```python
from build123d import *

# Parameters (mm, degrees)
SKETCH1_W           = 107.95
SKETCH1_H           = 101.6
BOSS_EXTRUDE1_DEPTH = 3.175
CUT_EXTRUDE1_REACH  = 5.175
SKETCH2_R           = 15.24
CUT_EXTRUDE2_REACH  = 5.175
SKETCH3_R           = 1.5875
CUT_EXTRUDE3_REACH  = 5.175
SKETCH4_R           = 2.1971
FILLET1_R           = 2.54
CUT_EXTRUDE4_DEPTH  = 4.175
FILLET3_R           = 0.0635


with BuildPart() as part:
    # Sketch1 → Boss-Extrude1 (new body)
    with BuildSketch(Plane.XY):
        with Locations((-16.095613336, 62.506086957)):
            Rectangle(SKETCH1_W, SKETCH1_H)
    extrude(amount=BOSS_EXTRUDE1_DEPTH)

    # Sketch2 → Cut-Extrude1 (cut, up to next)
    with BuildSketch(Plane.XY.offset(3.175), mode=Mode.PRIVATE) as cut_extrude1_sk1:
        with Locations((-16.095613336, 62.506086957)):
            Circle(SKETCH2_R)
    cut_extrude1_tool1 = extrude(cut_extrude1_sk1.sketch, amount=-CUT_EXTRUDE1_REACH, mode=Mode.PRIVATE) & part.part
    add(cut_extrude1_tool1.solids().sort_by_distance((-16.095613, 62.506087, 3.175))[0], mode=Mode.SUBTRACT)
    # Sketch2 → Cut-Extrude1 (cut, up to next)
    with BuildSketch(Plane.XY.offset(3.175), mode=Mode.PRIVATE) as cut_extrude1_sk2:
        with Locations((16.596179657, 32.989293963)):
            Circle(SKETCH2_R)
    cut_extrude1_tool2 = extrude(cut_extrude1_sk2.sketch, amount=-CUT_EXTRUDE1_REACH, mode=Mode.PRIVATE) & part.part
    add(cut_extrude1_tool2.solids().sort_by_distance((16.59618, 32.989294, 3.175))[0], mode=Mode.SUBTRACT)
    # Sketch2 → Cut-Extrude1 (cut, up to next)
    with BuildSketch(Plane.XY.offset(3.175), mode=Mode.PRIVATE) as cut_extrude1_sk3:
        with Locations((16.596179657, 92.02287995)):
            Circle(SKETCH2_R)
    cut_extrude1_tool3 = extrude(cut_extrude1_sk3.sketch, amount=-CUT_EXTRUDE1_REACH, mode=Mode.PRIVATE) & part.part
    add(cut_extrude1_tool3.solids().sort_by_distance((16.59618, 92.02288, 3.175))[0], mode=Mode.SUBTRACT)
    # Sketch2 → Cut-Extrude1 (cut, up to next)
    with BuildSketch(Plane.XY.offset(3.175), mode=Mode.PRIVATE) as cut_extrude1_sk4:
        with Locations((-48.787406329, 92.02287995)):
            Circle(SKETCH2_R)
    cut_extrude1_tool4 = extrude(cut_extrude1_sk4.sketch, amount=-CUT_EXTRUDE1_REACH, mode=Mode.PRIVATE) & part.part
    add(cut_extrude1_tool4.solids().sort_by_distance((-48.787406, 92.02288, 3.175))[0], mode=Mode.SUBTRACT)
    # Sketch2 → Cut-Extrude1 (cut, up to next)
    with BuildSketch(Plane.XY.offset(3.175), mode=Mode.PRIVATE) as cut_extrude1_sk5:
        with Locations((-48.787406329, 32.989293963)):
            Circle(SKETCH2_R)
    cut_extrude1_tool5 = extrude(cut_extrude1_sk5.sketch, amount=-CUT_EXTRUDE1_REACH, mode=Mode.PRIVATE) & part.part
    add(cut_extrude1_tool5.solids().sort_by_distance((-48.787406, 32.989294, 3.175))[0], mode=Mode.SUBTRACT)

    # Sketch3 → Cut-Extrude2 (cut, up to next)
    with BuildSketch(Plane.XY.offset(3.175), mode=Mode.PRIVATE) as cut_extrude2_sk1:
        with Locations((-31.186104332, 109.624181947)):
            Circle(SKETCH3_R)
    cut_extrude2_tool1 = extrude(cut_extrude2_sk1.sketch, amount=-CUT_EXTRUDE2_REACH, mode=Mode.PRIVATE) & part.part
    add(cut_extrude2_tool1.solids().sort_by_distance((-31.186104, 109.624182, 3.175))[0], mode=Mode.SUBTRACT)
    # Sketch3 → Cut-Extrude2 (cut, up to next)
    with BuildSketch(Plane.XY.offset(3.175), mode=Mode.PRIVATE) as cut_extrude2_sk2:
        with Locations((-66.388708326, 74.421577952)):
            Circle(SKETCH3_R)
    cut_extrude2_tool2 = extrude(cut_extrude2_sk2.sketch, amount=-CUT_EXTRUDE2_REACH, mode=Mode.PRIVATE) & part.part
    add(cut_extrude2_tool2.solids().sort_by_distance((-66.388708, 74.421578, 3.175))[0], mode=Mode.SUBTRACT)
    # Sketch3 → Cut-Extrude2 (cut, up to next)
    with BuildSketch(Plane.XY.offset(3.175), mode=Mode.PRIVATE) as cut_extrude2_sk3:
        with Locations((-1.00512234, 109.624181947)):
            Circle(SKETCH3_R)
    cut_extrude2_tool3 = extrude(cut_extrude2_sk3.sketch, amount=-CUT_EXTRUDE2_REACH, mode=Mode.PRIVATE) & part.part
    add(cut_extrude2_tool3.solids().sort_by_distance((-1.005122, 109.624182, 3.175))[0], mode=Mode.SUBTRACT)
    # Sketch3 → Cut-Extrude2 (cut, up to next)
    with BuildSketch(Plane.XY.offset(3.175), mode=Mode.PRIVATE) as cut_extrude2_sk4:
        with Locations((34.197481654, 74.421577952)):
            Circle(SKETCH3_R)
    cut_extrude2_tool4 = extrude(cut_extrude2_sk4.sketch, amount=-CUT_EXTRUDE2_REACH, mode=Mode.PRIVATE) & part.part
    add(cut_extrude2_tool4.solids().sort_by_distance((34.197482, 74.421578, 3.175))[0], mode=Mode.SUBTRACT)
    # Sketch3 → Cut-Extrude2 (cut, up to next)
    with BuildSketch(Plane.XY.offset(3.175), mode=Mode.PRIVATE) as cut_extrude2_sk5:
        with Locations((-31.186104332, 15.387991966)):
            Circle(SKETCH3_R)
    cut_extrude2_tool5 = extrude(cut_extrude2_sk5.sketch, amount=-CUT_EXTRUDE2_REACH, mode=Mode.PRIVATE) & part.part
    add(cut_extrude2_tool5.solids().sort_by_distance((-31.186104, 15.387992, 3.175))[0], mode=Mode.SUBTRACT)
    # Sketch3 → Cut-Extrude2 (cut, up to next)
    with BuildSketch(Plane.XY.offset(3.175), mode=Mode.PRIVATE) as cut_extrude2_sk6:
        with Locations((-66.388708326, 50.590595961)):
            Circle(SKETCH3_R)
    cut_extrude2_tool6 = extrude(cut_extrude2_sk6.sketch, amount=-CUT_EXTRUDE2_REACH, mode=Mode.PRIVATE) & part.part
    add(cut_extrude2_tool6.solids().sort_by_distance((-66.388708, 50.590596, 3.175))[0], mode=Mode.SUBTRACT)
    # Sketch3 → Cut-Extrude2 (cut, up to next)
    with BuildSketch(Plane.XY.offset(3.175), mode=Mode.PRIVATE) as cut_extrude2_sk7:
        with Locations((-1.00512234, 15.387991966)):
            Circle(SKETCH3_R)
    cut_extrude2_tool7 = extrude(cut_extrude2_sk7.sketch, amount=-CUT_EXTRUDE2_REACH, mode=Mode.PRIVATE) & part.part
    add(cut_extrude2_tool7.solids().sort_by_distance((-1.005122, 15.387992, 3.175))[0], mode=Mode.SUBTRACT)
    # Sketch3 → Cut-Extrude2 (cut, up to next)
    with BuildSketch(Plane.XY.offset(3.175), mode=Mode.PRIVATE) as cut_extrude2_sk8:
        with Locations((34.197481654, 50.590595961)):
            Circle(SKETCH3_R)
    cut_extrude2_tool8 = extrude(cut_extrude2_sk8.sketch, amount=-CUT_EXTRUDE2_REACH, mode=Mode.PRIVATE) & part.part
    add(cut_extrude2_tool8.solids().sort_by_distance((34.197482, 50.590596, 3.175))[0], mode=Mode.SUBTRACT)
    # Sketch3 → Cut-Extrude2 (cut, up to next)
    with BuildSketch(Plane.XY.offset(3.175), mode=Mode.PRIVATE) as cut_extrude2_sk9:
        with Locations((8.796386664, 62.506086957)):
            Circle(SKETCH3_R)
    cut_extrude2_tool9 = extrude(cut_extrude2_sk9.sketch, amount=-CUT_EXTRUDE2_REACH, mode=Mode.PRIVATE) & part.part
    add(cut_extrude2_tool9.solids().sort_by_distance((8.796387, 62.506087, 3.175))[0], mode=Mode.SUBTRACT)
    # Sketch3 → Cut-Extrude2 (cut, up to next)
    with BuildSketch(Plane.XY.offset(3.175), mode=Mode.PRIVATE) as cut_extrude2_sk10:
        with Locations((-40.987613336, 62.506086957)):
            Circle(SKETCH3_R)
    cut_extrude2_tool10 = extrude(cut_extrude2_sk10.sketch, amount=-CUT_EXTRUDE2_REACH, mode=Mode.PRIVATE) & part.part
    add(cut_extrude2_tool10.solids().sort_by_distance((-40.987613, 62.506087, 3.175))[0], mode=Mode.SUBTRACT)

    # Sketch4 → Cut-Extrude3 (cut, up to next)
    with BuildSketch(Plane.XY.offset(3.175), mode=Mode.PRIVATE) as cut_extrude3_sk1:
        with Locations((-16.095613336, 100.606086957)):
            Circle(SKETCH4_R)
    cut_extrude3_tool1 = extrude(cut_extrude3_sk1.sketch, amount=-CUT_EXTRUDE3_REACH, mode=Mode.PRIVATE) & part.part
    add(cut_extrude3_tool1.solids().sort_by_distance((-16.095613, 100.606087, 3.175))[0], mode=Mode.SUBTRACT)
    # Sketch4 → Cut-Extrude3 (cut, up to next)
    with BuildSketch(Plane.XY.offset(3.175), mode=Mode.PRIVATE) as cut_extrude3_sk2:
        with Locations((-16.095613336, 24.406086957)):
            Circle(SKETCH4_R)
    cut_extrude3_tool2 = extrude(cut_extrude3_sk2.sketch, amount=-CUT_EXTRUDE3_REACH, mode=Mode.PRIVATE) & part.part
    add(cut_extrude3_tool2.solids().sort_by_distance((-16.095613, 24.406087, 3.175))[0], mode=Mode.SUBTRACT)
    # Sketch4 → Cut-Extrude3 (cut, up to next)
    with BuildSketch(Plane.XY.offset(3.175), mode=Mode.PRIVATE) as cut_extrude3_sk3:
        with Locations((-54.195613336, 62.506086957)):
            Circle(SKETCH4_R)
    cut_extrude3_tool3 = extrude(cut_extrude3_sk3.sketch, amount=-CUT_EXTRUDE3_REACH, mode=Mode.PRIVATE) & part.part
    add(cut_extrude3_tool3.solids().sort_by_distance((-54.195613, 62.506087, 3.175))[0], mode=Mode.SUBTRACT)
    # Sketch4 → Cut-Extrude3 (cut, up to next)
    with BuildSketch(Plane.XY.offset(3.175), mode=Mode.PRIVATE) as cut_extrude3_sk4:
        with Locations((22.004386664, 62.506086957)):
            Circle(SKETCH4_R)
    cut_extrude3_tool4 = extrude(cut_extrude3_sk4.sketch, amount=-CUT_EXTRUDE3_REACH, mode=Mode.PRIVATE) & part.part
    add(cut_extrude3_tool4.solids().sort_by_distance((22.004387, 62.506087, 3.175))[0], mode=Mode.SUBTRACT)

    # Fillet1
    fillet1_edges = [part.edges().sort_by_distance(p)[0] for p in [
        (37.879386664, 11.706086957, 1.5875),
        (-70.070613336, 11.706086957, 1.5875),
        (-70.070613336, 113.306086957, 1.5875),
        (37.879386664, 113.306086957, 1.5875),
    ]]
    fillet(fillet1_edges, radius=FILLET1_R)

    # Sketch5 → Cut-Extrude4 (cut, through all)
    with BuildSketch(Plane.XY.offset(3.175)):
        Polygon((-64.355613336, 63.014086957), (-64.355613336, 61.998086957), (-65.625613336, 61.998086957), (-65.625613336, 61.490086957), (-66.895613336, 62.506086957), (-65.625613336, 63.522086957), (-65.625613336, 63.014086957), align=None)
    extrude(amount=-CUT_EXTRUDE4_DEPTH, mode=Mode.SUBTRACT)

    # Fillet3
    fillet3_edges = [part.edges().sort_by_distance(p)[0] for p in [
        (-65.625613336, 61.998086957, 1.5875),
        (-65.625613336, 61.490086957, 1.5875),
        (-66.895613336, 62.506086957, 1.5875),
        (-65.625613336, 63.522086957, 1.5875),
        (-65.625613336, 63.014086957, 1.5875),
        (-64.355613336, 63.014086957, 1.5875),
        (-64.355613336, 61.998086957, 1.5875),
    ]]
    fillet(fillet3_edges, radius=FILLET3_R)


solid = part.part
```
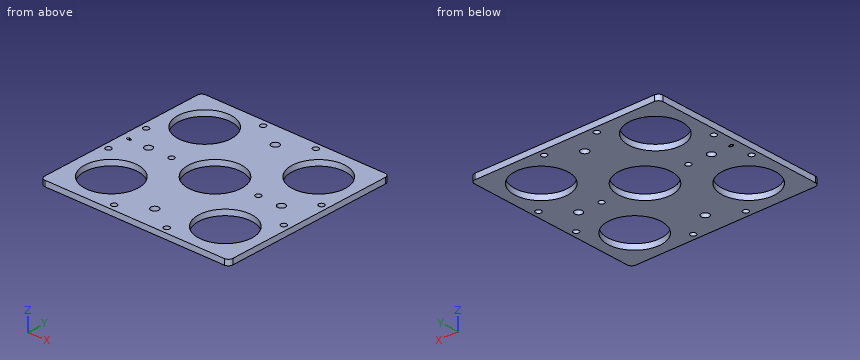
Geometry check sheet. Reference: the model listing, model coordinates, mm. Give positions to 0.01 mm unless a question says otherwise; leave off trailing zeros. Write each loop counter-clockwise with the first axis right and the second up, starting at its lowest first coordinate (ties: lowest second). Pieces come first, ordered by that corner, then holes. Notation, with made-up numbers: (29.25, 57.25) - (46.25, 57.25) arc R28 cw to (46.25, 78.25) - close; hole circle Ø3 at (60, -2.75). An arc over 180 degrees is marked (long way). Use a Markdown table: item, result.
Q1. Section check C-C, the plane y = 67. Enter the section's corners in (x, z) (3 decimals).
Computed:
| item | result |
|---|---|
| outline | (-70.071, 0) - (-30.658, 0) - (-30.658, 3.175) - (-70.071, 3.175) - close; (-1.533, 0) - (37.879, 0) - (37.879, 3.175) - (-1.533, 3.175) - close |
Q2. Thickness scan on L1, parallel to X at y = 92, z = 2.7; L2, parallel to Y at x = 16, z = 1.9; L3, parallel to X at y = 105, z = 0.25. Record the ranges inside material, lowest first. Write a range as [from, to].
Computed:
| item | result |
|---|---|
| L1 | x = [-70.07, -64.03], [-33.55, 1.36], [31.84, 37.88] |
| L2 | y = [11.71, 17.76], [48.22, 76.79], [107.25, 113.31] |
| L3 | x = [-70.07, -56.78], [-40.8, 8.61], [24.59, 37.88] |
Q3. Go/stop test with a flat-tipped pin: P1, Ø5.5, axis at x = -16.1, y = 100.61, coming from the +Z side (3 decimals). Record where the tip stops, or that it passes through.
Computed:
| item | result |
|---|---|
| P1 | stops at z = 3.175 |
Q4. Section check D-D, the plane x = -23. Enter the section's corners in (y, z) (3 decimals), then the cut area to 3 significant figures.
Computed:
| item | result |
|---|---|
| outline | (11.706, 0) - (48.92, 0) - (48.92, 3.175) - (11.706, 3.175) - close; (76.092, 0) - (113.306, 0) - (113.306, 3.175) - (76.092, 3.175) - close |
| area | 236 mm² |
Q5. Section check A-A, the plane x = -54.5. Enter the section's corners in (y, z) (3 decimals).
Computed:
| item | result |
|---|---|
| outline | (11.706, 0) - (18.86, 0) - (18.86, 3.175) - (11.706, 3.175) - close; (47.118, 0) - (60.33, 0) - (60.33, 3.175) - (47.118, 3.175) - close; (64.682, 0) - (77.894, 0) - (77.894, 3.175) - (64.682, 3.175) - close; (106.152, 0) - (113.306, 0) - (113.306, 3.175) - (106.152, 3.175) - close |
Q6. Section check B-B, the plane y = 28. Enter the section's corners in (x, z) (3 decimals), then the cut area to 3 significant figures.
Computed:
| item | result |
|---|---|
| outline | (-70.071, 0) - (-63.188, 0) - (-63.188, 3.175) - (-70.071, 3.175) - close; (-34.387, 0) - (2.196, 0) - (2.196, 3.175) - (-34.387, 3.175) - close; (30.996, 0) - (37.879, 0) - (37.879, 3.175) - (30.996, 3.175) - close |
| area | 160 mm² |
